from build123d import *
from build123d.topology import SkipClean

# Parameters (mm, degrees)
EXTRUDE_THIN1_DEPTH = 25
SKETCH3_R           = 2.25
BOSS_EXTRUDE1_DEPTH = 5


with BuildPart() as part:
    # Sketch2 → Extrude-Thin1 (new body)
    with BuildSketch(Plane(origin=(0, 0, 0), x_dir=(1, 0, 0), z_dir=(0, 1, 0))):
        with BuildLine():
            Line((-4, 52.659282183), (-4, 49))
            ThreePointArc((-4, 49), (0, 45), (4, 49))
            Line((4, 49), (4, 52.659282183))
            ThreePointArc((4, 52.659282183), (4.668239922, 54.151399837), (6.226415094, 54.646424907))
            ThreePointArc((6.226415094, 54.646424907), (47.631397208, 27.5), (50.438399742, -21.930978807))
            ThreePointArc((50.438399742, -21.930978807), (49.23060787, -23.032885555), (47.604276115, -22.865539476))
            Line((47.604276115, -22.865539476), (44.435244785, -21.035898385))
            ThreePointArc((44.435244785, -21.035898385), (38.97114317, -22.5), (40.435244785, -27.964101615))
            Line((40.435244785, -27.964101615), (43.604276115, -29.793742707))
            ThreePointArc((43.604276115, -29.793742707), (44.562367948, -31.118514282), (44.211984648, -32.7154461))
            ThreePointArc((44.211984648, -32.7154461), (0, -55), (-44.211984648, -32.715446099))
            ThreePointArc((-44.211984648, -32.715446099), (-44.562367948, -31.118514282), (-43.604276115, -29.793742706))
            Line((-43.604276115, -29.793742706), (-40.435244785, -27.964101615))
            ThreePointArc((-40.435244785, -27.964101615), (-38.97114317, -22.5), (-44.435244785, -21.035898385))
            Line((-44.435244785, -21.035898385), (-47.604276115, -22.865539476))
            ThreePointArc((-47.604276115, -22.865539476), (-49.23060787, -23.032885555), (-50.438399742, -21.930978807))
            ThreePointArc((-50.438399742, -21.930978807), (-47.631397208, 27.5), (-6.226415094, 54.646424907))
            ThreePointArc((-6.226415094, 54.646424907), (-4.668239922, 54.151399837), (-4, 52.659282183))
        make_face()
        with BuildLine():
            Line((-5.6, 52.659282183), (-5.6, 49))
            ThreePointArc((-5.6, 49), (0, 43.4), (5.6, 49))
            Line((5.6, 49), (5.6, 52.659282183))
            ThreePointArc((5.6, 52.659282183), (5.733647984, 52.957705714), (6.045283019, 53.056710728))
            ThreePointArc((6.045283019, 53.056710728), (46.245756562, 26.7), (48.971100841, -21.292986696))
            ThreePointArc((48.971100841, -21.292986696), (48.729542466, -21.513368046), (48.404276115, -21.47989883))
            Line((48.404276115, -21.47989883), (45.235244785, -19.650257739))
            ThreePointArc((45.235244785, -19.650257739), (37.585502524, -21.7), (39.635244785, -29.349742261))
            Line((39.635244785, -29.349742261), (42.804276115, -31.179383353))
            ThreePointArc((42.804276115, -31.179383353), (42.995894482, -31.444337668), (42.925817822, -31.763724031))
            ThreePointArc((42.925817822, -31.763724031), (0, -53.4), (-42.925817822, -31.763724031))
            ThreePointArc((-42.925817822, -31.763724031), (-42.995894482, -31.444337668), (-42.804276115, -31.179383353))
            Line((-42.804276115, -31.179383353), (-39.635244785, -29.349742261))
            ThreePointArc((-39.635244785, -29.349742261), (-37.585502524, -21.7), (-45.235244785, -19.650257739))
            Line((-45.235244785, -19.650257739), (-48.404276115, -21.47989883))
            ThreePointArc((-48.404276115, -21.47989883), (-48.729542466, -21.513368046), (-48.971100841, -21.292986696))
            ThreePointArc((-48.971100841, -21.292986696), (-46.245756562, 26.7), (-6.045283019, 53.056710728))
            ThreePointArc((-6.045283019, 53.056710728), (-5.733647984, 52.957705714), (-5.6, 52.659282183))
        make_face(mode=Mode.SUBTRACT)
    extrude(amount=EXTRUDE_THIN1_DEPTH)

    # Sketch3 → Boss-Extrude1 (add)
    # profile 1 of 3: a face of its own
    with SkipClean():  # the faces are left unmerged after this step: merging them gives an invalid solid
        with BuildSketch(Plane.XZ):
            with BuildLine():
                Line((-43.604276115, 29.793742706), (-40.435244785, 27.964101615))
                ThreePointArc((-40.435244785, 27.964101615), (-38.97114317, 22.5), (-44.435244785, 21.035898385))
                Line((-44.435244785, 21.035898385), (-47.604276115, 22.865539476))
                ThreePointArc((-47.604276115, 22.865539476), (-49.23060787, 23.032885555), (-50.438399742, 21.930978807))
                ThreePointArc((-50.438399742, 21.930978807), (-47.631397208, 27.5), (-44.211984648, 32.715446099))
                ThreePointArc((-44.211984648, 32.715446099), (-44.562367948, 31.118514282), (-43.604276115, 29.793742706))
            make_face()
            with Locations(Location((-42.435244785, 24.5, 0), (0, 0, 270))):
                Circle(SKETCH3_R, mode=Mode.SUBTRACT)
        # profile 2 of 3: a face of its own
        with BuildSketch(Plane.XZ):
            with BuildLine():
                Line((-4, -52.659282183), (-4, -49))
                ThreePointArc((-4, -49), (0, -45), (4, -49))
                Line((4, -49), (4, -52.659282183))
                ThreePointArc((4, -52.659282183), (4.668239922, -54.151399837), (6.226415094, -54.646424907))
                ThreePointArc((6.226415094, -54.646424907), (0, -55), (-6.226415094, -54.646424907))
                ThreePointArc((-6.226415094, -54.646424907), (-4.668239922, -54.151399837), (-4, -52.659282183))
            make_face()
            with Locations(Location((0, -49, 0), (0, 0, 270))):
                Circle(SKETCH3_R, mode=Mode.SUBTRACT)
        # profile 3 of 3: a face of its own
        with BuildSketch(Plane.XZ):
            with BuildLine():
                Line((47.604276115, 22.865539476), (44.435244785, 21.035898385))
                ThreePointArc((44.435244785, 21.035898385), (38.97114317, 22.5), (40.435244785, 27.964101615))
                Line((40.435244785, 27.964101615), (43.604276115, 29.793742707))
                ThreePointArc((43.604276115, 29.793742707), (44.562367948, 31.118514282), (44.211984648, 32.7154461))
                ThreePointArc((44.211984648, 32.7154461), (47.631397208, 27.5), (50.438399742, 21.930978807))
                ThreePointArc((50.438399742, 21.930978807), (49.23060787, 23.032885555), (47.604276115, 22.865539476))
            make_face()
            with Locations(Location((42.435244785, 24.5, 0), (0, 0, 270))):
                Circle(SKETCH3_R, mode=Mode.SUBTRACT)
        extrude(amount=-BOSS_EXTRUDE1_DEPTH)


solid = part.part
For this review, take the finished solid that the model builds, in its own axes (mm). A direction names the side the tool comes from. Round coordinates to 2 decimals unless told otherwise and drop trailing zeros. Order: outer loops, then holes, each group sorted by start corner. A loop starts at its lowest first (then second) coordinate and runs counter-clockwise, first axis right, second up. Notation, with made-up numbers: (74.5, 87.5) -> (114.5, 87.5) arc R25 ccw to (114.5, 126.5) -> close; hole circle Ø5 at (48.5, 43). An arc over 180 degrees is marked (long way). Write item = value, one per line. Start each with the question number.
1) Take a section at B-B on z = -4.5. State the section outline as (x, y) points.
2) Take a section at D-D on z = 24.5. State the section outline as (x, y) points.
3) Tool access review of faces 4 (the face through (-44, 5, 27)), 5 (the face through (-44.567, 14.86, 31.142)), 6 (the face through (45.893, 12.325, -27.302)): name each direction out of +Z, -Z, +X, -X, +Y, -Y from which nothing blocks a thin tool from reaching the whole face with its end or side.
4) Take a section at A-A on x = 0. State the section outline as (y, z) points.
5) The part is to be moulded in two halves that separate along Z. For faces 1 (the face through (4, 15, -51)), 2 (the face through (37.65, 12.32, 21.59)), 3 (the face through (0, 15, -45)), say which applies: +Z half, -Z half, draft (parallel to the pull), parting line (faces both ways), or undercut.
6) Insertion check: pin 1 (3.5 mm diameter, centred on x = 44.5, z = 25.5, fed in from +Y); pin 2 (6 mm diameter, centred on y = 15, z = 28, fed in from -X); pin 3 (4 mm diameter, centred on x = -11, y = 5.5, fed in from -Z); pin 4 (4 mm diameter, centred on x = 0, z = -49, fed in from -Y). Each pin has a flat end and moves straight along its axis. Give the tip position at first contact, or say it passes through.
7) To check wall thickness, follow line 1 (X direction, y = 2.6, z = -49); line 2 (Z direction, x = 37.5, y = 11); line 3 (X direction, y = 1.4, z = 24.5). State the ranges of each line that lie inside material, in increasing order. Write a range as from..to.
8) Take a section at C-C on x = -19. State the section outline as (y, z) points.
Verdict:
q1.outline = (-54.82, 0) -> (-53.21, 0) -> (-53.21, 25) -> (-54.82, 25) -> close; (53.21, 0) -> (54.82, 0) -> (54.82, 25) -> (53.21, 25) -> close
q2.outline = (-49.24, 0) -> (-44.69, 0) -> (-44.69, 5) -> (-49.24, 5) -> close; (-40.19, 0) -> (-36.84, 0) -> (-36.84, 25) -> (-38.44, 25) -> (-38.44, 5) -> (-40.19, 5) -> close; (36.84, 0) -> (40.19, 0) -> (40.19, 5) -> (38.44, 5) -> (38.44, 25) -> (36.84, 25) -> close; (44.69, 0) -> (49.24, 0) -> (49.24, 5) -> (44.69, 5) -> close
q3.face_4 = +Y
q3.face_5 = -X, +Y
q3.face_6 = +Y, -Y
q4.outline = (0, -55) -> (5, -55) -> (5, -51.25) -> (0, -51.25) -> close; (0, -46.75) -> (5, -46.75) -> (5, -45) -> (25, -45) -> (25, -43.4) -> (0, -43.4) -> close; (0, 53.4) -> (25, 53.4) -> (25, 55) -> (0, 55) -> close
q5.face_1 = draft
q5.face_2 = undercut
q5.face_3 = -Z half
q6.pin_1 = 5
q6.pin_2 = -44.53
q6.pin_3 = -54.26
q6.pin_4 = through
q7.line_1 = -24.98..-21.23, -5.6..-2.25, 2.25..5.6, 21.23..24.98
q7.line_2 = -40.23..-38.02, 21.85..27.15, 38.02..40.23
q7.line_3 = -49.24..-44.69, -40.19..-36.84, 36.84..40.19, 44.69..49.24
q8.outline = (0, -51.61) -> (25, -51.61) -> (25, -49.91) -> (0, -49.91) -> close; (0, 49.91) -> (25, 49.91) -> (25, 51.61) -> (0, 51.61) -> close
